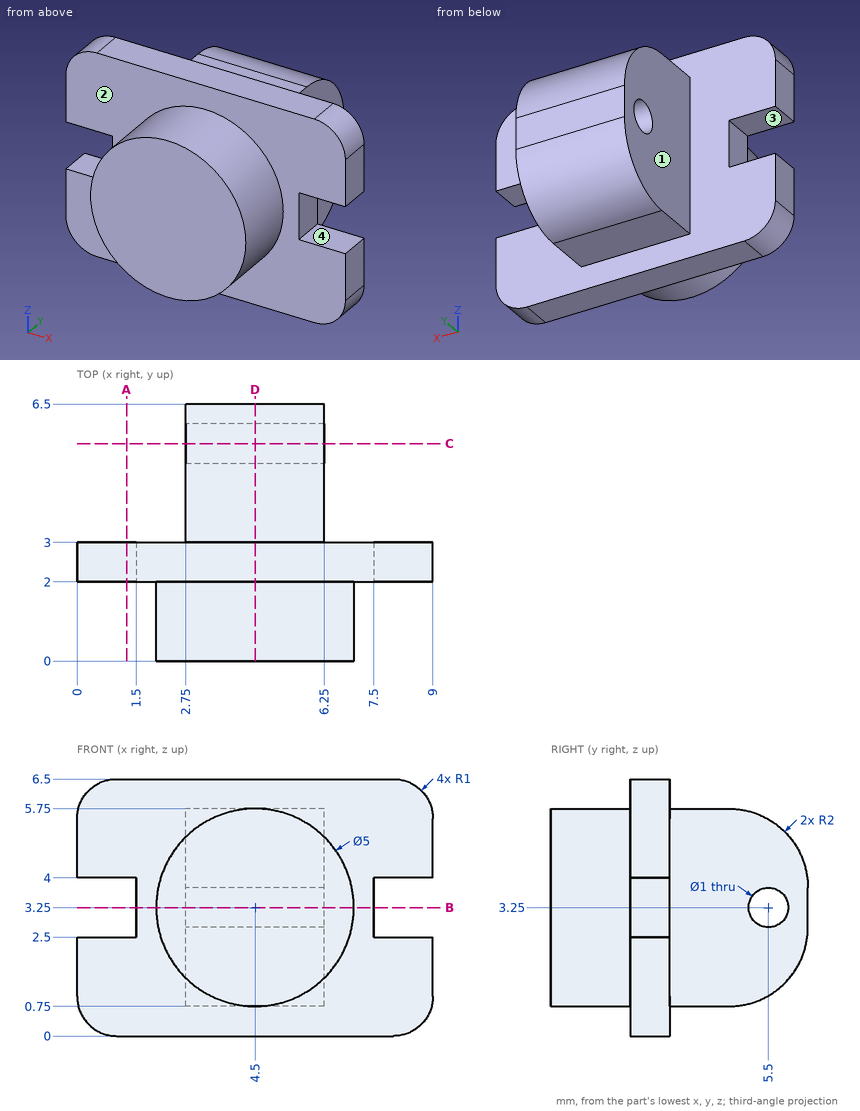
The drawing under review shows one solid part. Ordinate dimensions are in mm from its lowest x, y, z. A direction names the side the tool comes from. Coordinates: 2 decimals unless noted, no trailing zeros. Write each loop counter-clockwise with the first axis right and the second up, starting at its lowest first coordinate (ties: lowest second). Pieces come first, ordered by that corner, then holes. Notation, with made-up numbers: (-13.75, -12) - (19.25, -12) arc R22 cw to (19.25, 13) - close; hole circle Ø8 at (40.25, 6). An arc over 180 degrees is marked (long way). Answer in a Markdown table with one row per item. Add a question column.
Q1. We need section B-B, the plane z = 3.25. State the section outline as (x, y) points.
Q2. For probe 1 along Y at (x, z) = (0.5, 4.25); probe 2 along Z at (x, y) = (5.55, 5.5); probe 3 along X at (y, z) = (5.25, 4.25), list the stretches that pass through material, from the lowest coordinate up.
Q3. Tool access review of the marked faces 1, 2, 3 and 4: name each direction out of +Z, -Z, +X, -X, +Y, -Y from which nothing blocks a thin tool from reaching the whole face with its end or side.
Q4. We need section D-D, the plane x = 4.5. State the section outline as (y, z) points.
Q5. For P1, Ø2, axis at x = 6, z = 2, coming from the +Y side; P2, Ø0.5, axis at y = 2.5, z = 3.5, coming from the +X side; P3, Ø1.8, axis at y = 5, z = 2, coming from the -X side; P4, Ø0.5, axis at x = 8.5, y = 2.5, coming from the +Z side, all flat-tipped, find the tip position at first contact; note any pin that passes through.
Q6. We need section C-C, the plane y = 5.5. State the section outline as (x, z) points, and give its area (3 significant figures).
Q7. We need section A-A, the plane x = 1.25. State the section outline as (y, z) points.
Answer list:
| question | item | result |
|---|---|---|
| 1 | outline | (1.5, 2) - (2, 2) - (2, 0) - (7, 0) - (7, 2) - (7.5, 2) - (7.5, 3) - (6.25, 3) - (6.25, 5) - (2.75, 5) - (2.75, 3) - (1.5, 3) - close; (2.75, 6) - (6.25, 6) - (6.25, 6.5) - (2.75, 6.5) - close |
| 2 | probe 1 | y = 2 to 3 |
| 2 | probe 2 | z = 1.02 to 2.75, 3.75 to 5.48 |
| 2 | probe 3 | x = 2.75 to 6.25 |
| 3 | face 1 | +Z, -Z, -X, +Y |
| 3 | face 2 | -Y |
| 3 | face 3 | -X, +Y, -Y |
| 3 | face 4 | +X, +Y, -Y |
| 4 | outline | (0, 0.75) - (2, 0.75) - (2, 0) - (3, 0) - (3, 0.75) - (4.5, 0.75) arc R2 ccw to (6.5, 2.75) - (6.5, 3.75) arc R2 ccw to (4.5, 5.75) - (3, 5.75) - (3, 6.5) - (2, 6.5) - (2, 5.75) - (0, 5.75) - close; hole circle Ø1 at (5.5, 3.25) |
| 5 | P1 | stops at y = 6.5 |
| 5 | P2 | stops at x = 7.5 |
| 5 | P3 | stops at x = 2.75 |
| 5 | P4 | stops at z = 6.47 |
| 6 | outline | (2.75, 1.02) - (6.25, 1.02) - (6.25, 2.75) - (2.75, 2.75) - close; (2.75, 3.75) - (6.25, 3.75) - (6.25, 5.48) - (2.75, 5.48) - close |
| 6 | area | 12.1 mm2 |
| 7 | outline | (2, 0) - (3, 0) - (3, 2.5) - (2, 2.5) - close; (2, 4) - (3, 4) - (3, 6.5) - (2, 6.5) - close |
